Geometry: final body of the model. Coordinates: model frame, mm. Face numbers are marked on the shaded views. A direction names the side the tool comes from. Give positions to 0.01 mm unless a question says otherwise; leave off trailing zeros. Write each loop counter-clockwise with the first axis right and the second up, starting at its lowest first coordinate (ties: lowest second). Pieces come first, ordered by that corner, then holes. Notation, with made-up numbers: (72, 21) - (113, 21) arc R14 ccw to (113, 33) - close; hole circle Ø3 at (83.25, 0.25). An arc over 180 degrees is marked (long way). Use CSV: the item, a comma, the result in double quotes. Start each with the question number.
(1) Reachability of the marked faces 4 and 5 from +Z, -Z, +X, -X, +Y, -Y: full face, straight path, thin tool, end or side. Return the list, or none.
(2) Draft query along Z for the marked faces 1, 2 and 3. Return one class per face: released by +Z, released by -Z, zero draft, split by the parting line, or undercut.
(3) Section B-B on z = -6.5. Output: boundary loops of the cut face in (x, y).
(4) First-contact query: pin 1 Ø1.2 at (y, z) = (257.5, 324) entering from -X; pin 2 Ø10 at (x, z) = (-49.5, -61) entering from -Y; pin 3 Ø1 at (x, y) = (-36.5, 172.5) entering from -Z. Flat tips, straight axial feed; report the tip coordinate or a pass-through.
(5) Line query: probe 1 along Z at (x, y) = (-9.5, 139.5); probe 2 along Z at (x, y) = (-22.5, 194.5); probe 3 along Y at (x, z) = (-42, 178). Output: solid intervals per line, ascending. Write a range as [from, to].
(6) Section A-A on y = 179.5. Output: boundary loops of the cut face in (x, z).
from build123d import *

# Parameters (mm, degrees)
BASE_FLANGE1_DEPTH       = 347
EDGE_FLANGE1_DEPTH       = 255.5
SKETCH5_W                = 301.8
SKETCH5_H                = 83
CUT_EXTRUDE1_DEPTH       = 10
SKETCH6_W                = 41.9
SKETCH6_H                = 45.9
CUT_EXTRUDE2_DEPTH       = 1.5
CUT_EXTRUDE3_DEPTH       = 1.5
EDGE_FLANGE2_DEPTH       = 255.5
M5_START                 = 349.3
M5_CLEARANCE_SLOT1_DEPTH = 1.5
FILLET1_R                = 5
M5_START_2               = 257
M5_CLEARANCE_SLOT2_DEPTH = 1.5
FILLET2_R                = 5
FILLET3_R                = 3
SKETCH15_W               = 96
SKETCH15_H               = 68
CUT_EXTRUDE4_DEPTH       = 10
SKETCH16_W               = 85
SKETCH16_H               = 68
CUT_EXTRUDE5_DEPTH       = 1.5
FILLET4_R                = 5
FILLET5_R                = 3
CUT_EXTRUDE6_DEPTH       = 750.483248688
CUT_EXTRUDE6_DEPTH_BACK  = 4
FILLET6_R                = 5


# Read off the part's stored shape, not the designer's step: M5 Clearance Slot1, M5 Clearance Slot2
# Sheet-metal steps are written as plain solids
with BuildPart() as part:
    # Sketch1 → Base-Flange1 (new, symmetric)
    with BuildSketch(Plane.XY):
        with BuildLine():
            Line((-61.5, 258.5), (-3, 258.5))
            ThreePointArc((-3, 258.5), (-0.878679656, 257.621320344), (0, 255.5))
            Line((0, 255.5), (0, 0))
            Line((0, 0), (-1.5, 0))
            Line((-1.5, 0), (-1.5, 255.5))
            ThreePointArc((-1.5, 255.5), (-1.939339828, 256.560660172), (-3, 257))
            Line((-3, 257), (-61.5, 257))
            Line((-61.5, 257), (-61.5, 258.5))
        make_face()
    extrude(amount=BASE_FLANGE1_DEPTH, both=True)

    # Edge-Flange1 section (across the edge) → Edge-Flange1 (add)
    with BuildSketch(Plane(origin=(-1.5, 0, 349.3), x_dir=(0, 0, -1), z_dir=(0, 1, 0))):
        with BuildLine():
            Line((-1.5, 1.5), (-1.5, 60))
            Line((-1.5, 60), (0, 60))
            Line((0, 60), (0, 1.5))
            ThreePointArc((0, 1.5), (0.439339828, 0.439339828), (1.5, 0))
            Line((1.5, 0), (2.3, 0))
            Line((2.3, 0), (2.3, -1.5))
            Line((2.3, -1.5), (1.5, -1.5))
            ThreePointArc((1.5, -1.5), (-0.621320344, -0.621320344), (-1.5, 1.5))
        make_face()
    extrude(amount=EDGE_FLANGE1_DEPTH)

    # Sketch5 → Cut-Extrude1 (cut)
    with BuildSketch(Plane(origin=(0, 0, 0), x_dir=(0, 0, -1), z_dir=(1, 0, 0))):
        with Locations((-24.9, 41.5)):
            Rectangle(SKETCH5_W, SKETCH5_H)
    extrude(amount=-CUT_EXTRUDE1_DEPTH, mode=Mode.SUBTRACT)

    # Sketch6 → Cut-Extrude2 (cut)
    with BuildSketch(Plane(origin=(0, 258.5, 0), x_dir=(1, 0, 0), z_dir=(0, 1, 0))):
        with Locations((-40.55, 324.05)):
            Rectangle(SKETCH6_W, SKETCH6_H)
    extrude(amount=-CUT_EXTRUDE2_DEPTH, mode=Mode.SUBTRACT)

    # Sketch7 → Cut-Extrude3 (cut)
    with BuildSketch(Plane(origin=(0, 258.5, 0), x_dir=(1, 0, 0), z_dir=(0, 1, 0))):
        with BuildLine():
            Line((-40.3, -335), (-40.3, -303))
            ThreePointArc((-40.3, -303), (-42.643145751, -297.343145751), (-48.3, -295))
            Line((-48.3, -295), (-71.165008453, -295))
            Line((-71.165008453, -295), (-71.165008453, -343))
            Line((-71.165008453, -343), (-71.165008453, -364.064767585))
            Line((-71.165008453, -364.064767585), (-40.3, -364.064767585))
            Line((-40.3, -364.064767585), (-40.3, -335))
        make_face()
    extrude(amount=-CUT_EXTRUDE3_DEPTH, mode=Mode.SUBTRACT)

    # Edge-Flange2 section (across the edge) → Edge-Flange2 (add)
    with BuildSketch(Plane(origin=(-1.5, 255.5, -348.5), x_dir=(0, 0, 1), z_dir=(0, -1, 0))):
        with BuildLine():
            Line((-1.5, 1.5), (-1.5, 18.1))
            Line((-1.5, 18.1), (0, 18.1))
            Line((0, 18.1), (0, 1.5))
            ThreePointArc((0, 1.5), (0.439339828, 0.439339828), (1.5, 0))
            Line((1.5, 0), (1.5, -1.5))
            ThreePointArc((1.5, -1.5), (-0.621320344, -0.621320344), (-1.5, 1.5))
        make_face()
    extrude(amount=EDGE_FLANGE2_DEPTH)

    # M5 Clearance Slot1 outline → M5 Clearance Slot1 (cut)
    with BuildSketch(Plane.XY.offset(M5_START)):
        with BuildLine():
            Line((-61.5, 42.1), (-51.4, 42.1))
            ThreePointArc((-51.4, 42.1), (-48.5, 45), (-51.4, 47.9))
            Line((-51.4, 47.9), (-61.5, 47.9))
            Line((-61.5, 47.9), (-61.5, 42.1))
        make_face()
        with BuildLine():
            Line((-61.5, 202.9), (-61.5, 197.1))
            Line((-61.5, 197.1), (-51.4, 197.1))
            ThreePointArc((-51.4, 197.1), (-48.5, 200), (-51.4, 202.9))
            Line((-51.4, 202.9), (-61.5, 202.9))
        make_face()
    extrude(amount=M5_CLEARANCE_SLOT1_DEPTH, mode=Mode.SUBTRACT)

    # Fillet1
    fillet1_edges = [part.edges().sort_by_distance(p)[0] for p in [
        (-61.5, 42.1, 350.05),
        (-61.5, 47.9, 350.05),
        (-61.5, 197.1, 350.05),
        (-61.5, 202.9, 350.05),
        (-61.5, 0, 350.05),
        (-61.5, 255.5, 350.05),
    ]]
    fillet(fillet1_edges, radius=FILLET1_R)

    # M5 Clearance Slot2 outline → M5 Clearance Slot2 (cut)
    with BuildSketch(Plane(origin=(0, 0, 0), x_dir=(1, 0, 0), z_dir=(0, 1, 0)).offset(M5_START_2)):
        with BuildLine():
            Line((-51, 191.9), (-61.2, 191.9))
            ThreePointArc((-61.2, 191.9), (-61.350201599, 191.896107643), (-61.5, 191.88444102))
            Line((-61.5, 191.88444102), (-61.5, 186.11555898))
            ThreePointArc((-61.5, 186.11555898), (-61.350201599, 186.103892357), (-61.2, 186.1))
            Line((-61.2, 186.1), (-51, 186.1))
            ThreePointArc((-51, 186.1), (-48.1, 189), (-51, 191.9))
        make_face()
        with BuildLine():
            ThreePointArc((-61.2, -186.1), (-61.350201599, -186.103892357), (-61.5, -186.11555898))
            Line((-61.5, -186.11555898), (-61.5, -191.88444102))
            ThreePointArc((-61.5, -191.88444102), (-61.350201599, -191.896107643), (-61.2, -191.9))
            Line((-61.2, -191.9), (-51, -191.9))
            ThreePointArc((-51, -191.9), (-48.1, -189), (-51, -186.1))
            Line((-51, -186.1), (-61.2, -186.1))
        make_face()
    extrude(amount=M5_CLEARANCE_SLOT2_DEPTH, mode=Mode.SUBTRACT)

    # Fillet2
    fillet2_edges = [part.edges().sort_by_distance(p)[0] for p in [
        (-61.5, 257.75, 186.11555898),
        (-61.5, 257.75, 191.88444102),
        (-61.5, 257.75, -191.88444102),
        (-61.5, 257.75, -186.11555898),
    ]]
    fillet(fillet2_edges, radius=FILLET2_R)

    # Fillet3
    fillet3_edges = [part.edges().sort_by_distance(p)[0] for p in [
        (-19.6, 255.5, -349.25),
        (-19.6, 0, -349.25),
        (-19.6, 257.75, -347),
    ]]
    fillet(fillet3_edges, radius=FILLET3_R)

    # Sketch15 → Cut-Extrude4 (cut)
    with BuildSketch(Plane(origin=(0, 0, 0), x_dir=(0, 0, -1), z_dir=(1, 0, 0))):
        with Locations((174, 34)):
            Rectangle(SKETCH15_W, SKETCH15_H)
    extrude(amount=-CUT_EXTRUDE4_DEPTH, mode=Mode.SUBTRACT)

    # Sketch16 → Cut-Extrude5 (cut)
    with BuildSketch(Plane(origin=(0, 0, 0), x_dir=(0, 0, -1), z_dir=(1, 0, 0))):
        with Locations((-218.3, 34)):
            Rectangle(SKETCH16_W, SKETCH16_H)
    extrude(amount=-CUT_EXTRUDE5_DEPTH, mode=Mode.SUBTRACT)

    # Fillet4
    fillet4_edges = [part.edges().sort_by_distance(p)[0] for p in [
        (-0.75, 68, -126),
        (-0.75, 68, -222),
        (-0.75, 68, 175.8),
        (-0.75, 68, 260.8),
        (-0.75, 83, 175.8),
        (-0.75, 83, -126),
    ]]
    fillet(fillet4_edges, radius=FILLET4_R)

    # Fillet5
    fillet5_edges = [part.edges().sort_by_distance(p)[0] for p in [
        (-40.3, 257.75, 347),
        (-61.5, 257.75, 295),
    ]]
    fillet(fillet5_edges, radius=FILLET5_R)

    # Sketch17 → Cut-Extrude6 (cut, two sides: drawn at the far end of the back side and taken through both)
    with BuildSketch(Plane.XY.offset(350.8).offset(-CUT_EXTRUDE6_DEPTH_BACK)):
        with BuildLine():
            Line((-61.5, 250.5), (-61.5, 237.5))
            Line((-61.5, 237.5), (-41.5, 237.5))
            ThreePointArc((-41.5, 237.5), (-37.964466094, 238.964466094), (-36.5, 242.5))
            Line((-36.5, 242.5), (-36.5, 255.5))
            Line((-36.5, 255.5), (-56.5, 255.5))
            ThreePointArc((-56.5, 255.5), (-60.035533906, 254.035533906), (-61.5, 250.5))
        make_face()
    extrude(amount=CUT_EXTRUDE6_DEPTH + CUT_EXTRUDE6_DEPTH_BACK, mode=Mode.SUBTRACT)

    # Fillet6
    fillet6_edges = [part.edges().sort_by_distance(p)[0] for p in [
        (-61.5, 237.5, 350.05),
        (-36.5, 255.5, 350.05),
    ]]
    fillet(fillet6_edges, radius=FILLET6_R)


solid = part.part
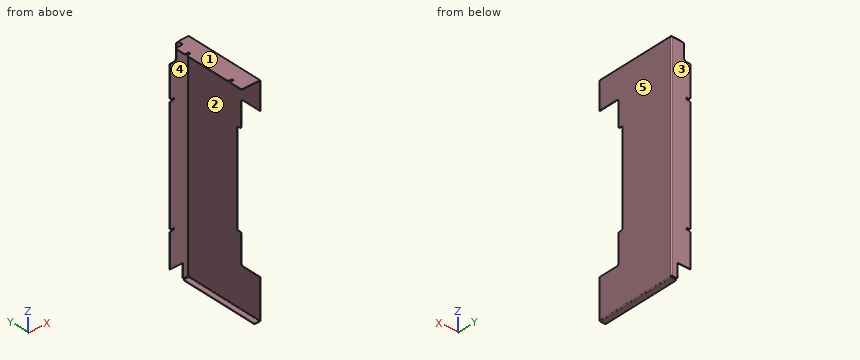
Check values:
1,face 4,"+Z, -Z, -X, -Y"
1,face 5,"+Z, -Z, +X, +Y, -Y"
2,face 1,"released by +Z"
2,face 2,"undercut"
2,face 3,"zero draft"
3,outline,"(-61.5, 257) - (-3, 257) arc R1.5 cw to (-1.5, 255.5) - (-1.5, 83) - (0, 83) - (0, 255.5) arc R3 ccw to (-3, 258.5) - (-61.5, 258.5) - close"
4,pin 1,"stops at x = -40.3"
4,pin 2,"stops at y = 257"
4,pin 3,"stops at z = 349.3"
5,probe 1,"z = [-350, -348.5], [349.3, 350.8]"
5,probe 2,"z = [349.3, 350.8]"
5,probe 3,"y = [257, 258.5]"
6,outline,"(-61.5, 349.3) - (-3, 349.3) arc R1.5 cw to (-1.5, 347.8) - (-1.5, -347) arc R1.5 cw to (-3, -348.5) - (-19.6, -348.5) - (-19.6, -350) - (-3, -350) arc R3 ccw to (0, -347) - (0, 347.8) arc R3 ccw to (-3, 350.8) - (-61.5, 350.8) - close"
